Geometry: final body of the model. Coordinates: model frame, mm. Round coordinates to 2 decimals unless told otherwise and drop trailing zeros. Order: outer loops, then holes, each group sorted by start corner. A loop starts at its lowest first (then second) coordinate and runs counter-clockwise, first axis right, second up. Notation, with made-up numbers: M -31,2.5 L -1,2.5 A21 cw -1,22.5 Z; hole C -38.5,54 d4. An arc over 180 degrees is marked long. Return JSON: item names as keys, results as strings. Group by question number.
Q1. Contact query for flat-ended pins moving along their axis: pin 1 (4 mm diameter, centred on x = 6, y = -5, fed in from +Z); pin 2 (10 mm diameter, centred on x = 2, y = 10.5, fed in from +Z). Output: stop coordinate, or through.
Q2. Ray query, probe 1 along Z at (x, y) = (-5, -1.5); probe 2 along X at (y, z) = (-14.5, 375). Return the intervals inside material, ascending.
Q3. Cut plane B-B on z = 461.5. Output: boundary loops of the cut face in (x, y).
Q4. Cut plane C-C on y = 5.5. Output: boundary loops of the cut face in (x, z), and give its area (3 significant figures).
Q5. Cut plane A-A on x = 0. Output: boundary loops of the cut face in (y, z) (3 decimals), and give its area (3 significant figures).
```python
from build123d import *

# Parameters (mm, degrees)
F1_DEPTH = 1063.625
F3_DEPTH = 38.1


with BuildPart() as f1:
    # F0 (on Top) → F1 (new body)
    with BuildSketch(Plane.XY):
        with BuildLine():
            ThreePointArc((19.05, 12.7), (17.1901280605, 17.1901280605), (12.7, 19.05))
            Line((12.7, 19.05), (-12.7, 19.05))
            ThreePointArc((-12.7, 19.05), (-17.1901280605, 17.1901280605), (-19.05, 12.7))
            Line((-19.05, 12.7), (-19.05, -12.7))
            ThreePointArc((-19.05, -12.7), (-17.1901280605, -17.1901280605), (-12.7, -19.05))
            Line((-12.7, -19.05), (12.7, -19.05))
            ThreePointArc((12.7, -19.05), (17.1901280605, -17.1901280605), (19.05, -12.7))
            Line((19.05, -12.7), (19.05, 12.7))
        make_face()
    extrude(amount=F1_DEPTH)

    # F2 (on face) → F3 (cut)
    with BuildSketch(Plane(origin=(-19.05, 0, 0), x_dir=(0, -1, 0), z_dir=(-1, 0, 0))):
        Polygon((12.7, 1063.625), (12.7, 1008.6323868597), (19.05, 997.6338642316), (19.05, 1063.625), align=None)
        Polygon((-12.7, 1063.625), (-12.7, 1052.6264773719), (12.7, 1008.6323868597), (12.7, 1063.625), align=None)
        Polygon((-12.7, 1063.625), (-19.05, 1063.625), (-12.7, 1052.6264773719), align=None)
    extrude(amount=-F3_DEPTH, mode=Mode.SUBTRACT)


solid = f1.part
```
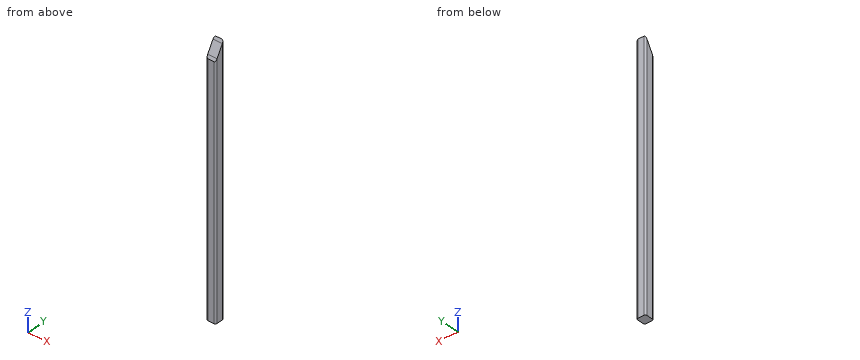
Result sheet:
{
 "1": {"pin 1": "stops at z = 1025.43", "pin 2": "stops at z = 1057.48"},
 "2": {"probe 1": "z = 0 to 1028.03", "probe 2": "x = -18.79 to 18.79"},
 "3": {"outline": "M -19.05,-12.7 A6.35 ccw -12.7,-19.05 L 12.7,-19.05 A6.35 ccw 19.05,-12.7 L 19.05,12.7 A6.35 ccw 12.7,19.05 L -12.7,19.05 A6.35 ccw -19.05,12.7 Z"},
 "4": {"outline": "M -19.05,0 L 19.05,0 L 19.05,1040.16 L -19.05,1040.16 Z", "area": "39,600 mm²"},
 "5": {"outline": "M -19.05,0 L 19.05,0 L 19.05,1063.625 L -19.05,997.634 Z", "area": "39,300 mm²"}
}
